Input: part model. Units: mm. Frame: model coordinates. A direction names the side the tool comes from. Round coordinates to 2 decimals unless told otherwise and drop trailing zeros. Order: outer loops, then holes, each group sorted by start corner. A loop starts at its lowest first (then second) coordinate and runs counter-clockwise, first axis right, second up. Notation, with made-up numbers: M 81,63 L 125,63 A20 cw 125,68 Z; hole C -10,42 d7. An arc over 180 degrees is marked long. One line per question, with ' | ' between items.
```python
from build123d import *

# Parameters (mm, degrees)
SKETCH1_W           = 20
SKETCH1_H           = 30
BOSS_EXTRUDE1_DEPTH = 6
SKETCH2_R           = 1.72792937
CUT_EXTRUDE1_DEPTH  = 7
CUT_EXTRUDE2_DEPTH  = 3


with BuildPart() as part:
    # Sketch1 → Boss-Extrude1 (new body)
    with BuildSketch(Plane.XY):
        with Locations((10, 15)):
            Rectangle(SKETCH1_W, SKETCH1_H)
    extrude(amount=BOSS_EXTRUDE1_DEPTH)

    # Sketch2 → Cut-Extrude1 (cut, through all)
    with BuildSketch(Plane.XY.offset(6)):
        with Locations((15.5, 23.816694008)):
            Circle(SKETCH2_R)
        with Locations((3.5, 20.102573312)):
            Circle(SKETCH2_R)
        with Locations((17.55, 5.5)):
            Circle(SKETCH2_R)
        with Locations((3.45, 8.361159496)):
            Circle(SKETCH2_R)
    extrude(amount=-CUT_EXTRUDE1_DEPTH, mode=Mode.SUBTRACT)

    # Sketch3 → Cut-Extrude2 (cut)
    with BuildSketch(Plane.XY.offset(6)):
        Polygon((20, 26.616694008), (13.683419246, 26.616694008), (12.066838493, 23.816694008), (13.683419246, 21.016694008), (20, 21.016694008), align=None)
        Polygon((6.933161507, 20.102573312), (5.316580754, 22.902573312), (0, 22.902573312), (0, 17.302573312), (5.316580754, 17.302573312), align=None)
        Polygon((6.883161507, 8.361159496), (5.266580754, 11.161159496), (0, 11.161159496), (0, 5.561159496), (5.266580754, 5.561159496), align=None)
        Polygon((14.116838493, 5.5), (15.733419246, 2.7), (20, 2.7), (20, 8.3), (15.733419246, 8.3), align=None)
    extrude(amount=-CUT_EXTRUDE2_DEPTH, mode=Mode.SUBTRACT)


solid = part.part
```
Item 1: First-contact query: pin 1 (3.5 mm diameter, centred on x = 3, z = 5, fed in from -Y); pin 2 (2 mm diameter, centred on x = 3.5, y = 20.1, fed in from -Z); pin 3 (5.5 mm diameter, centred on x = 3.45, y = 8.36, fed in from +Z). Flat tips, straight axial feed; report the tip coordinate or a pass-through.
Report:
pin 1: y = 0 | pin 2: through | pin 3: z = 3
Item 2: Section query D-D, the plane x = 3.5. Return loops of the section in (y, z).
Report:
outline: M 0,0 L 6.63,0 L 6.63,3 L 5.56,3 L 5.56,6 L 0,6 Z; M 10.09,0 L 18.37,0 L 18.37,3 L 17.3,3 L 17.3,6 L 11.16,6 L 11.16,3 L 10.09,3 Z; M 21.83,0 L 30,0 L 30,6 L 22.9,6 L 22.9,3 L 21.83,3 Z
Item 3: Line query: line 1 along Y through (x, z) = (3.75, 4.7); line 2 along Y through (x, z) = (3.5, 0.8); line 3 along Y through (x, z) = (15.5, 1.6). Output: solid intervals per line, ascending. Write a range as from..to.
Report:
line 1: 0..5.56, 11.16..17.3, 22.9..30 | line 2: 0..6.63, 10.09..18.37, 21.83..30 | line 3: 0..22.09, 25.54..30
Item 4: Section query A-A, the plane z = 0.9. Return loops of the section in (x, y), plus the area to 3 significant figures.
Report:
outline: M 0,0 L 20,0 L 20,30 L 0,30 Z; hole C 3.45,8.36 d3.46; hole C 3.5,20.1 d3.46; hole C 15.5,23.82 d3.46; hole C 17.55,5.5 d3.46 | area: 562 mm²
Item 5: Section query C-C, the plane y = 20.5. Return loops of the section in (x, z), plus the area to 3 significant figures.
Report:
outline: M 0,0 L 1.82,0 L 1.82,3 L 0,3 Z; M 5.18,0 L 20,0 L 20,6 L 6.7,6 L 6.7,3 L 5.18,3 Z | area: 89.8 mm²
Item 6: Section query B-B, the plane x = 17.55. Return loops of the section in (y, z), plus the area to 3 significant figures.
Report:
outline: M 0,0 L 3.77,0 L 3.77,3 L 2.7,3 L 2.7,6 L 0,6 Z; M 7.23,0 L 30,0 L 30,6 L 26.62,6 L 26.62,3 L 21.02,3 L 21.02,6 L 8.3,6 L 8.3,3 L 7.23,3 Z | area: 136 mm²
Item 7: Mould query, pull axis X, two halves, no side actions, for faces 4 (the flat face through (12.86, 22.44, 4.52)), 5 (the cylindrical face through (3.075, 6.674, 1.521)), 6 (the flat face through (10, 15, 0)). Classes: +X half, -X half, draft (parallel to the pull), parting line (faces both ways), or undercut.
Report:
face 4: +X half | face 5: undercut | face 6: draft
Item 8: Access query for faces 1 (the flat face through (6.11, 18.68, 4.52)), 2 (the flat face through (17, 26.617, 5)), 3 (the cylindrical face through (17.175, 3.813, 1.521)). Directions: +Z, -Z, +X, -X, +Y, -Y. A direction counts if a zero-diameter tool reaches every point of the face in a straight line with its end or side. Return the directions, or none.
Report:
face 1: +Z, -X | face 2: +Z, +X | face 3: +Z, -Z
